Design review of the part built by this model. Coordinates are the model's own, in mm. A direction names the side the tool comes from. Round coordinates to 2 decimals unless told otherwise and drop trailing zeros. Loops run counter-clockwise (first coordinate to the right, second up) from the corner with the lowest first, then second, coordinate; pieces in that order, holes last. Notation, with made-up numbers: (12.5, 18) - (71.5, 18) arc R19 ccw to (71.5, 49) - close; hole circle Ø8 at (83, 48). An arc over 180 degrees is marked (long way). Return JSON: item names as keys, results as strings. Group by question number.
(1) Clearance check with flat-ended pins moving along their axes: pin 1 (4 mm diameter, centred on x = 47, z = 42, fed in from +Y); pin 2 (6 mm diameter, centred on y = 53.5, z = 87, fed in from -X); pin 3 (12 mm diameter, centred on x = 31, z = 26.5, fed in from -Y). State where each tip first meets the part, or that it passes through.
(2) We need section A-A, the plane z = 105.5. Write out the cut boundary in (x, y).
(3) For faces 4 (the cylindrical face through (118.02, 115.45, 77.09)), 5 (the flat face through (186, 186, 139.7)), 6 (the flat face through (185, 196, 146.05)), 7 (the flat face through (131, 131, 0)), list the 3-axis set-ups (+Z, -Z, +X, -X, +Y, -Y) from which the entire face can be reached by the end or side of a thin tool; tool diameter is ignored.
(4) The part is to be moulded in two halves that separate along Y. For faces 1 (the cylindrical face through (113.48, 111.01, 75.31)), 2 (the flat face through (127, 131, 6.35)), 3 (the flat face through (129, 129, 146.05)), say which applies: pulls with the +Y half, pulls with the -Y half, needs draft (parallel to the pull), parting line crosses it, or undercut.
(5) Wall thickness on L1, parallel to Z at x = 152.5, y = 167; L2, parallel to Z at x = 172.5, y = 205; L3, parallel to Z at x = 207, y = 154.5: over which ranges is each line inside the solid? List them lowest first. Write a range as [from, to].
from build123d import *

# Parameters (mm, degrees)
F1_ANGLE = 90


# Not quite as in the source:
# - ends of sketch curves that miss each other by under 0.0002 mm in the source are joined


with BuildPart() as f1:
    # F0 (on Front) → F1 (revolve)
    with BuildSketch(Plane.XZ):
        with BuildLine():
            Line((158.75, 139.7), (158.75, 12.7))
            ThreePointArc((158.75, 12.7), (162.4697438789, 3.7197438789), (171.45, 0))
            Line((171.45, 0), (257.81, 0))
            ThreePointArc((257.81, 0), (259.6060512242, 0.7439487758), (260.35, 2.54))
            Line((260.35, 2.54), (260.35, 3.8099999233))
            ThreePointArc((260.35, 3.8099999233), (259.6060512242, 5.6060511475), (257.81, 6.3499999233))
            Line((257.81, 6.3499999233), (171.45, 6.3499999233))
            ThreePointArc((171.45, 6.3499999233), (166.9598694704, 8.2098694704), (165.0999965083, 12.7))
            Line((165.0999965083, 12.7), (165.1, 139.7))
            ThreePointArc((165.1, 139.7), (166.9598719395, 144.1901280605), (171.45, 146.05))
            Line((171.45, 146.05), (254.3705810057, 146.05))
            ThreePointArc((254.3705810057, 146.05), (257.5772088315, 141.4621426782), (262.89, 139.7))
            Line((262.89, 139.7), (270.51, 139.7))
            ThreePointArc((270.51, 139.7), (272.3060512242, 140.4439487758), (273.05, 142.24))
            Line((273.05, 142.24), (273.05, 143.51))
            ThreePointArc((273.05, 143.51), (272.3060512242, 145.3060512242), (270.51, 146.05))
            Line((270.51, 146.05), (262.89, 146.05))
            ThreePointArc((262.89, 146.05), (261.0939487758, 146.7939487758), (260.35, 148.59))
            Line((260.35, 148.59), (260.35, 149.86))
            ThreePointArc((260.35, 149.86), (259.6060512242, 151.6560512242), (257.81, 152.4))
            Line((257.81, 152.4), (171.45, 152.4))
            ThreePointArc((171.45, 152.4), (162.4697438789, 148.6802561211), (158.75, 139.7))
        make_face()
    revolve(axis=Axis((0, 0, 68.397693336), (0, 0, 1)), revolution_arc=F1_ANGLE)


solid = f1.part
Solutions:
{
 "1": {"pin 1": "y = 158.85", "pin 2": "x = 148.36", "pin 3": "y = 154.38"},
 "2": {"outline": "(0, 158.75) arc R158.75 cw to (158.75, 0) - (165.1, 0) arc R165.1 ccw to (0, 165.1) - close"},
 "3": {"face 4": "+X, +Y", "face 5": "-Z, +X, +Y", "face 6": "+Z, +X, +Y", "face 7": "-Z, +X, -X, +Y, -Y"},
 "4": {"face 1": "pulls with the -Y half", "face 2": "needs draft", "face 3": "undercut"},
 "5": {"L1": "[0, 6.35], [146.05, 152.4]", "L2": "[139.7, 146.05]", "L3": "[0.05, 6.3], [140.98, 152.35]"}
}
